```python
from build123d import *

# Parameters (mm, degrees)
PAD024_DEPTH         = 80
PAD024_DEPTH_BACK    = 78
SKETCH039_R          = 2.1
PAD025_DEPTH         = 3
POCKET015_DEPTH      = 26.4508304953
POCKET015_DEPTH_BACK = 15.001


with BuildPart() as part:
    # Sketch038 → Pad024 (new body, two sides)
    with BuildSketch(Plane.XZ) as pad024_sk:
        Polygon((0, 15), (40, 15), (40, 5), (60, 5), (60, 0), (80, 0), (80, 5), (140, 5), (140, 2), (83, 2), (83, -3), (57, -3), (57, 2), (37, 2), (37, 12), (0, 12), align=None)
    extrude(amount=PAD024_DEPTH)
    extrude(pad024_sk.sketch, amount=-PAD024_DEPTH_BACK)

    # Sketch039 (on Face17 of Pad024) → Pad025 (join)
    with BuildSketch(Plane(origin=(0, 78, 0), x_dir=(1, 0, 0), z_dir=(0, 1, 0))):
        Polygon((140, -5), (140, 20.112497453), (117.0808832189, 12.2596635501), (112.2188710769, 26.4498304953), (0, -12), (0, -15), (40, -15), (40, -5), (60, -5), (60, 0), (80, 0), (80, -5), align=None)
        with Locations((131.5386824304, 4)):
            Circle(SKETCH039_R, mode=Mode.SUBTRACT)
        with Locations((111.4048164409, 10.3148586933)):
            Circle(SKETCH039_R, mode=Mode.SUBTRACT)
        with Locations((108.1634750128, 19.7749699901)):
            Circle(SKETCH039_R, mode=Mode.SUBTRACT)
        with Locations((91.7780816016, 14.1608019521)):
            Circle(SKETCH039_R, mode=Mode.SUBTRACT)
        with Locations((101.5914490212, 12.2378303227)):
            Circle(SKETCH039_R, mode=Mode.SUBTRACT)
    extrude(amount=-PAD025_DEPTH)

    # Sketch048 → Pocket015 (cut, two sides)
    with BuildSketch(Plane.XY) as pocket015_sk:
        with BuildLine():
            ThreePointArc((7.9, -5), (10, -7.1), (12.1, -5))
            Line((12.1, -5), (12.1, 65))
            ThreePointArc((12.1, 65), (10, 67.1), (7.9, 65))
            Line((7.9, 65), (7.9, -5))
        make_face()
        with BuildLine():
            ThreePointArc((12.1, -15), (10, -12.9), (7.9, -15))
            Line((7.9, -15), (7.9, -70))
            ThreePointArc((7.9, -70), (10, -72.1), (12.1, -70))
            Line((12.1, -70), (12.1, -15))
        make_face()
        with BuildLine():
            ThreePointArc((27.9, -70), (30, -72.1), (32.1, -70))
            Line((32.1, -70), (32.1, -15))
            ThreePointArc((32.1, -15), (30, -12.9), (27.9, -15))
            Line((27.9, -15), (27.9, -70))
        make_face()
        with BuildLine():
            ThreePointArc((52.1, -5), (50, -2.9), (47.9, -5))
            Line((47.9, -5), (47.9, -60))
            ThreePointArc((47.9, -60), (50, -62.1), (52.1, -60))
            Line((52.1, -60), (52.1, -5))
        make_face()
        with BuildLine():
            ThreePointArc((67.9, -55), (70, -57.1), (72.1, -55))
            Line((72.1, -55), (72.1, 0))
            ThreePointArc((72.1, 0), (70, 2.1), (67.9, 0))
            Line((67.9, 0), (67.9, -55))
        make_face()
        with BuildLine():
            ThreePointArc((87.9, -68), (90, -70.1), (92.1, -68))
            Line((92.1, -68), (92.1, -5))
            ThreePointArc((92.1, -5), (90, -2.9), (87.9, -5))
            Line((87.9, -5), (87.9, -68))
        make_face()
        with BuildLine():
            ThreePointArc((112.1, -5), (110, -2.9), (107.9, -5))
            Line((107.9, -5), (107.9, -68))
            ThreePointArc((107.9, -68), (110, -70.1), (112.1, -68))
            Line((112.1, -68), (112.1, -5))
        make_face()
        with BuildLine():
            ThreePointArc((127.9, -68), (130, -70.1), (132.1, -68))
            Line((132.1, -68), (132.1, -5))
            ThreePointArc((132.1, -5), (130, -2.9), (127.9, -5))
            Line((127.9, -5), (127.9, -68))
        make_face()
        with BuildLine():
            ThreePointArc((127.9, 5), (130, 2.9), (132.1, 5))
            Line((132.1, 5), (132.1, 65))
            ThreePointArc((132.1, 65), (130, 67.1), (127.9, 65))
            Line((127.9, 65), (127.9, 5))
        make_face()
        with BuildLine():
            ThreePointArc((112.1, 65), (110, 67.1), (107.9, 65))
            Line((107.9, 65), (107.9, 5))
            ThreePointArc((107.9, 5), (110, 2.9), (112.1, 5))
            Line((112.1, 5), (112.1, 65))
        make_face()
        with BuildLine():
            ThreePointArc((87.9, 5), (90, 2.9), (92.1, 5))
            Line((92.1, 5), (92.1, 65))
            ThreePointArc((92.1, 65), (90, 67.1), (87.9, 65))
            Line((87.9, 65), (87.9, 5))
        make_face()
        with BuildLine():
            ThreePointArc((67.9, 10), (70, 7.9), (72.1, 10))
            Line((72.1, 10), (72.1, 65))
            ThreePointArc((72.1, 65), (70, 67.1), (67.9, 65))
            Line((67.9, 65), (67.9, 10))
        make_face()
        with BuildLine():
            ThreePointArc((47.9, 5), (50, 2.9), (52.1, 5))
            Line((52.1, 5), (52.1, 65))
            ThreePointArc((52.1, 65), (50, 67.1), (47.9, 65))
            Line((47.9, 65), (47.9, 5))
        make_face()
        with BuildLine():
            ThreePointArc((27.9, -5), (30, -7.1), (32.1, -5))
            Line((32.1, -5), (32.1, 65))
            ThreePointArc((32.1, 65), (30, 67.1), (27.9, 65))
            Line((27.9, 65), (27.9, -5))
        make_face()
    extrude(amount=-POCKET015_DEPTH, mode=Mode.SUBTRACT)
    extrude(pocket015_sk.sketch, amount=POCKET015_DEPTH_BACK, mode=Mode.SUBTRACT)


solid = part.part
```
Geometry: final body of the model. Coordinates: model frame, mm. A direction names the side the tool comes from. Give positions to 0.01 mm unless a question says otherwise; leave off trailing zeros. Loops run counter-clockwise (first coordinate to the right, second up) from the corner with the lowest first, then second, coordinate; pieces in that order, holes last. Notation, with made-up numbers: (-21, 11) -> (-16, 11) arc R18 cw to (-16, 39) -> close; hole circle Ø6 at (49.5, 4). An arc over 180 degrees is marked (long way). Return JSON: item names as keys, results as strings.
Item 1: Mould query, pull axis Z, two halves, no side actions, for faces 5 (the flat face through (60, -2, 3)), 6 (the cylindrical face through (103.594, 76.521, -12.869)), 7 (the flat face through (128.7, 76.52, -16.24)). Classes: released by +Z, released by -Z, zero draft, split by the parting line, or undercut.
Filled in:
{"face 5": "zero draft", "face 6": "undercut", "face 7": "released by -Z"}
Item 2: Section B-B, the plane y = 17. Count the separate pieces of the cut face and the enclosed holes in it, plus the area to 3 significant figures.
Filled in:
{"separate pieces": "8", "enclosed holes": "0", "area": "392 mm^2"}
Item 3: Access query for faces 1 (the flat face through (111.9, -3.6, 2)), 2 (the flat face through (73, -4, -3)), 3 (the flat face through (80, -2, 2)), 4 (the flat face through (114.684, 76.521, -19.255)). Directions: +Z, -Z, +X, -X, +Y, -Y. A direction counts if a zero-diameter tool reaches every point of the face in a straight line with its end or side. Return the directions, or none.
Filled in:
{"face 1": "-Z, +X, -Y", "face 2": "-Z, +X, -X, -Y", "face 3": "+Z, +Y, -Y", "face 4": "-Z, +Y, -Y"}
Item 4: Section A-A, the plane x = 50. Output: boundary loops of the cut face in (y, z).
Filled in:
{"outline": "(-80, 2) -> (-62.1, 2) -> (-62.1, 5) -> (-80, 5) -> close; (-2.9, 2) -> (2.9, 2) -> (2.9, 5) -> (-2.9, 5) -> close; (67.1, 2) -> (75, 2) -> (75, -5.13) -> (78, -5.13) -> (78, 5) -> (67.1, 5) -> close"}
Item 5: Pin query (flat end, axial travel): P1, Ø3, axis at x = 62.5, z = -12.5, coming from the +Y side; P2, Ø2, axis at x = 68, y = -19.5, coming from the -Z side; P3, Ø16, axis at x = 54.5, y = -26.5, coming from the +Z side; P4, Ø3.5, axis at y = -51, z = 14, coming from the +X side. Return the tip coordinate at first contact, or that it passes through.
Filled in:
{"P1": "through", "P2": "z = -3", "P3": "z = 5", "P4": "x = 40"}
Item 6: Section D-D, the plane x = 15.5. Output: boundary loops of the cut face in (y, z).
Filled in:
{"outline": "(-80, 12) -> (75, 12) -> (75, 6.69) -> (78, 6.69) -> (78, 15) -> (-80, 15) -> close"}
Item 7: Line query: line 1 (Z direction, x = 102, y = -67); line 2 (X direction, y = -72.5, z = 9); line 3 (Y direction, x = 94.5, z = -1.5). Output: solid intervals per line, ascending.
Filled in:
{"line 1": "2 to 5", "line 2": "37 to 40", "line 3": "75 to 78"}
Item 8: Section C-C, the plane z = 9. Output: boundary loops of the cut face in (x, y).
Filled in:
{"outline": "(8.76, 75) -> (37, 75) -> (37, -80) -> (40, -80) -> (40, 78) -> (8.76, 78) -> close"}
